from build123d import *

# Parameters (mm, degrees)
SKETCH1_R            = 24.5
BOSS_EXTRUDE1_DEPTH  = 2.54
M3_CLEARANCE_HOLE1_D = 3.4
SKETCH4_R            = 17.5
CUT_EXTRUDE1_DEPTH   = 1.27
SKETCH5_W            = 7.5
SKETCH5_H            = 7.5
CUT_EXTRUDE2_DEPTH   = 1.27


with BuildPart() as part:
    # Sketch1 → Boss-Extrude1 (new body)
    with BuildSketch(Plane(origin=(0, 0, 0), x_dir=(1, 0, 0), z_dir=(0, 1, 0))):
        with Locations(Location((0, 0, 0), (0, 0, 270))):
            Circle(SKETCH1_R)
    extrude(amount=BOSS_EXTRUDE1_DEPTH)

    # M3 Clearance Hole1 (through all)
    with Locations(Plane(origin=(-18.40303983, 2.54, 10.625), x_dir=(0, 0, 1), z_dir=(0, 1, 0))):
        with Locations((0, 0), (0, 36.80607966), (-31.875, 18.40303983)):
            Hole(M3_CLEARANCE_HOLE1_D / 2)

    # Sketch4 → Cut-Extrude1 (cut)
    with BuildSketch(Plane(origin=(0, 2.54, 0), x_dir=(1, 0, 0), z_dir=(0, 1, 0))):
        with Locations(Location((0, 0, 0), (0, 0, 270))):
            Circle(SKETCH4_R)
    extrude(amount=-CUT_EXTRUDE1_DEPTH, mode=Mode.SUBTRACT)

    # Sketch5 → Cut-Extrude2 (cut)
    with BuildSketch(Plane(origin=(0, 1.27, 0), x_dir=(1, 0, 0), z_dir=(0, 1, 0))):
        Rectangle(SKETCH5_W, SKETCH5_H)
    extrude(amount=-CUT_EXTRUDE2_DEPTH, mode=Mode.SUBTRACT)


solid = part.part
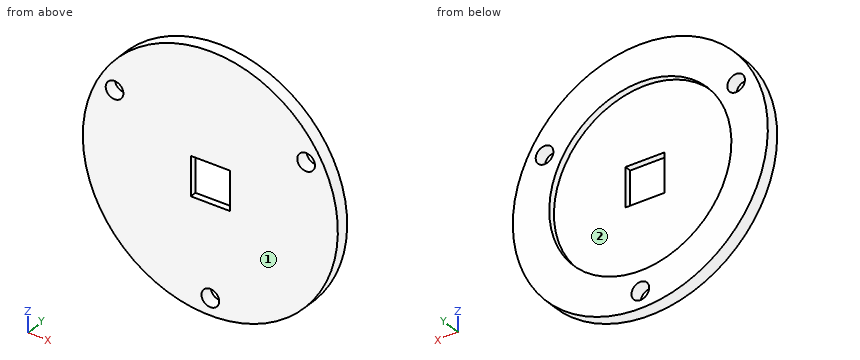
Work out the finished part from the listing and answer in its coordinate system (mm). Face numbers are marked on the shaded views. Coordinates: 2 decimals unless noted, no trailing zeros. Loops run counter-clockwise (first coordinate to the right, second up) from the corner with the lowest first, then second, coordinate; pieces in that order, holes last. Notation, with made-up numbers: M 68,66.25 L 115,66.25 A17 ccw 115,89.25 Z; hole C 50.25,78 d2. An arc over 180 degrees is marked long. Answer in a Markdown table with one row per item. Add a question column.
1. The mould has two halves that part along Z. Classify the marked faces 1 and 2: pulls with the +Z half, pulls with the -Z half, needs draft (parallel to the pull), parting line crosses it, or undercut.
2. Flat-ended cylindrical pins translate along their axes: P1, Ø3, axis at x = -2.5, z = 0, coming from the +Y side; P2, Ø0.6, axis at x = -0.5, y = 1, coming from the -Z side; P3, Ø1, axis at y = 1, z = 5.5, coming from the -X side; P4, Ø3, axis at x = -18.4, z = 10.62, coming from the -Y side. Find the tip coordinate at first contact, or state that the pin passes through.
3. Consider L1, parallel to X at y = 2.05, z = 0; L2, parallel to X at y = 2.3, z = 6; L3, parallel to Y at x = -5, z = 0. Determine where each line is inside the solid, lowest interval first.
4. Find section C-C, the plane y = 1.95. Write down the section's boundary in (x, z) (3 decimals), then the cut area to 3 significant figures.
5. Find section D-D, the plane x = -12. Write down the section's boundary in (y, z), then the cut area to 3 significant figures.
6. Find section B-B, the plane z = 0. Write down the section's boundary in (x, y).
7. Find section A-A, the plane x = 0. Write down the section's boundary in (y, z), then the cut area to 3 significant figures.
Reported:
| question | item | result |
|---|---|---|
| 1 | face 1 | needs draft |
| 1 | face 2 | undercut |
| 2 | P1 | stops at y = 1.27 |
| 2 | P2 | stops at z = -24.5 |
| 2 | P3 | stops at x = -23.98 |
| 2 | P4 | passes through |
| 3 | L1 | x = -24.5 to -17.5, 17.5 to 24.5 |
| 3 | L2 | x = -23.75 to -16.44, 16.44 to 23.75 |
| 3 | L3 | y = 0 to 1.27 |
| 4 | outline | C 0,0 d49; hole C -18.403,10.625 d3.4; hole C 0,0 d35; hole C 0,-21.25 d3.4; hole C 18.403,10.625 d3.4 |
| 4 | area | 896 mm^2 |
| 5 | outline | M 0,-21.36 L 2.54,-21.36 L 2.54,-12.74 L 1.27,-12.74 L 1.27,12.74 L 2.54,12.74 L 2.54,21.36 L 0,21.36 Z |
| 5 | area | 76.2 mm^2 |
| 6 | outline | M -24.5,0 L -3.75,0 L -3.75,1.27 L -17.5,1.27 L -17.5,2.54 L -24.5,2.54 Z; M 3.75,0 L 24.5,0 L 24.5,2.54 L 17.5,2.54 L 17.5,1.27 L 3.75,1.27 Z |
| 7 | outline | M 0,-24.5 L 2.54,-24.5 L 2.54,-22.95 L 0,-22.95 Z; M 0,-19.55 L 2.54,-19.55 L 2.54,-17.5 L 1.27,-17.5 L 1.27,-3.75 L 0,-3.75 Z; M 0,3.75 L 1.27,3.75 L 1.27,17.5 L 2.54,17.5 L 2.54,24.5 L 0,24.5 Z |
| 7 | area | 61.8 mm^2 |
